```python
from build123d import *

# Parameters (mm, degrees)
SKETCH1_R           = 9
BOSS_EXTRUDE1_DEPTH = 25
SKETCH3_R           = 10
BOSS_EXTRUDE2_DEPTH = 2
SKETCH4_R           = 9
BOSS_EXTRUDE3_DEPTH = 2
SKETCH5_R           = 10
BOSS_EXTRUDE4_DEPTH = 2
SKETCH6_R           = 9
BOSS_EXTRUDE5_DEPTH = 19
SKETCH7_R           = 8
CUT_EXTRUDE1_DEPTH  = 2
SKETCH8_R           = 1.5
BOSS_EXTRUDE6_DEPTH = 2
BOSS_EXTRUDE7_DEPTH = 2


with BuildPart() as part:
    # Sketch1 → Boss-Extrude1 (new body)
    with BuildSketch(Plane.XY):
        Circle(SKETCH1_R)
    extrude(amount=BOSS_EXTRUDE1_DEPTH)

    # Sketch3 → Boss-Extrude2 (add)
    with BuildSketch(Plane.XY.offset(25)):
        Circle(SKETCH3_R)
    extrude(amount=BOSS_EXTRUDE2_DEPTH)

    # Sketch4 → Boss-Extrude3 (add)
    with BuildSketch(Plane.XY.offset(27)):
        Circle(SKETCH4_R)
    extrude(amount=BOSS_EXTRUDE3_DEPTH)

    # Sketch5 → Boss-Extrude4 (add)
    with BuildSketch(Plane.XY.offset(29)):
        Circle(SKETCH5_R)
    extrude(amount=BOSS_EXTRUDE4_DEPTH)

    # Sketch6 → Boss-Extrude5 (add)
    with BuildSketch(Plane.XY.offset(31)):
        Circle(SKETCH6_R)
    extrude(amount=BOSS_EXTRUDE5_DEPTH)

    # Sketch7 → Cut-Extrude1 (cut)
    with BuildSketch(Plane.XY.offset(50)):
        Circle(SKETCH7_R)
    extrude(amount=-CUT_EXTRUDE1_DEPTH, mode=Mode.SUBTRACT)

    # Sketch8 → Boss-Extrude6 (add)
    with BuildSketch(Plane.XY.offset(48)):
        with Locations((-3.354571174, 0)):
            Circle(SKETCH8_R)
        with Locations((3.262554329, 0)):
            Circle(SKETCH8_R)
    extrude(amount=BOSS_EXTRUDE6_DEPTH)

    # Sketch9 → Boss-Extrude7 (add)
    with BuildSketch(Plane(origin=(0, 0, 0), x_dir=(-1, 0, 0), z_dir=(0, 0, -1))):
        with BuildLine():
            Line((2.630574057, 5.182535367), (6.058172796, 0.703309821))
            ThreePointArc((6.058172796, 0.703309821), (5.842389235, -0.919093383), (4.219986031, -0.703309821))
            Line((4.219986031, -0.703309821), (0.792387292, 3.775915724))
            ThreePointArc((0.792387292, 3.775915724), (1.008170853, 5.398318928), (2.630574057, 5.182535367))
        make_face()
    extrude(amount=BOSS_EXTRUDE7_DEPTH)


solid = part.part
```
Source: CAD feature listing. Evaluate the final solid. Frame: model axes, mm. A direction names the side the tool comes from. Coordinates: 2 decimals unless noted, no trailing zeros. Order: outer loops, then holes, each group sorted by start corner. A loop starts at its lowest first (then second) coordinate and runs counter-clockwise, first axis right, second up. Notation, with made-up numbers: (73, -24.75) - (84, -24.75) arc R8 cw to (84, -9.75) - close; hole circle Ø8 at (-4, 86.5). An arc over 180 degrees is marked (long way). One line per item, written item: value.
1) Cut plane B-B on z = 22.5. Output: boundary loops of the cut face in (x, y).
Computed values:
outline: circle Ø18 at (0, 0)
2) Cut plane D-D on x = -5.5. Output: boundary loops of the cut face in (y, z), plus the area to 3 significant figures.
Computed values:
outline: (-8.35, 25) - (-7.12, 25) - (-7.12, 0) - (-1.1, 0) - (-1.1, -2) - (1.43, -2) - (1.43, 0) - (7.12, 0) - (7.12, 25) - (8.35, 25) - (8.35, 27) - (7.12, 27) - (7.12, 29) - (8.35, 29) - (8.35, 31) - (7.12, 31) - (7.12, 50) - (5.81, 50) - (5.81, 48) - (-5.81, 48) - (-5.81, 50) - (-7.12, 50) - (-7.12, 31) - (-8.35, 31) - (-8.35, 29) - (-7.12, 29) - (-7.12, 27) - (-8.35, 27) - close
area: 704 mm^2
3) Cut plane A-A on x = 0. Output: boundary loops of the cut face in (y, z), plus the area to 3 significant figures.
Computed values:
outline: (-10, 25) - (-9, 25) - (-9, 0) - (9, 0) - (9, 25) - (10, 25) - (10, 27) - (9, 27) - (9, 29) - (10, 29) - (10, 31) - (9, 31) - (9, 50) - (8, 50) - (8, 48) - (-8, 48) - (-8, 50) - (-9, 50) - (-9, 31) - (-10, 31) - (-10, 29) - (-9, 29) - (-9, 27) - (-10, 27) - close
area: 876 mm^2
4) Contact query for flat-ended pins moving along their axis: pin 1 (12 mm diameter, centred on x = 7.5, y = 1.5, fed in from -Z); pin 2 (6 mm diameter, centred on y = 1, z = 40, fed in from +X); pin 3 (6 mm diameter, centred on x = -3, z = 39.5, fed in from -Y). Output: stop coordinate, or through.
Computed values:
pin 1: stops at z = 0
pin 2: stops at x = 9
pin 3: stops at y = -9
5) Reachability of faces 1 (the face through (-1.172, 8.923, 27.986)), 2 (the face through (-5.862, -0.903, -0.986)), 3 (the face through (-4.3, 3, -1)), 4 (the face through (-1.172, 8.923, 40.367)) from +Z, -Z, +X, -X, +Y, -Y: full face, straight path, thin tool, end or side. Return the list, or none.
Computed values:
face 1: none
face 2: -Z
face 3: -Z, -X, +Y
face 4: +Z
6) Cut plane C-C on y = -4.25. Output: boundary loops of the cut face in (x, z), plus the area to 3 significant figures.
Computed values:
outline: (-9.05, 25) - (-7.93, 25) - (-7.93, 0) - (7.93, 0) - (7.93, 25) - (9.05, 25) - (9.05, 27) - (7.93, 27) - (7.93, 29) - (9.05, 29) - (9.05, 31) - (7.93, 31) - (7.93, 50) - (6.78, 50) - (6.78, 48) - (-6.78, 48) - (-6.78, 50) - (-7.93, 50) - (-7.93, 31) - (-9.05, 31) - (-9.05, 29) - (-7.93, 29) - (-7.93, 27) - (-9.05, 27) - close
area: 775 mm^2
7) Mould query, pull axis Y, two halves, no side actions, for faces 5 (the face through (-3, 2, -2)), 6 (the face through (-1.172, 8.923, 12.325)), 7 (the face through (0, 0, 48)), 8 (the face through (-1.924, 0.451, 48.986)). Classes: released by +Y, released by -Y, zero draft, split by the parting line, or undercut.
Computed values:
face 5: zero draft
face 6: split by the parting line
face 7: undercut
face 8: undercut
8) Ray query, line 1 (Y direction, x = 0, z = 48.75); line 2 (Z direction, x = -1.5, y = 4.25); line 3 (Z direction, x = -5.75, y = 6.75). Return the intervals inside material, ascending. Write a range as [from, to].
Computed values:
line 1: y = [-9, -8], [8, 9]
line 2: z = [-2, 48]
line 3: z = [0, 50]
